The model under review builds one solid part; all positions refer to its coordinate system, in mm. A direction names the side the tool comes from. Coordinates: 2 decimals unless noted, no trailing zeros. Loops run counter-clockwise (first coordinate to the right, second up) from the corner with the lowest first, then second, coordinate; pieces in that order, holes last. Notation, with made-up numbers: (43, 37) - (65, 37) arc R29 ccw to (65, 74) - close; hole circle Ø2 at (60.5, 72). An arc over 180 degrees is marked (long way). Answer in a Markdown table with one row per item. Add a question column.
(1) We need section C-C on y = 63. Write out the cut boundary in (x, z), plus the area to 3 significant figures.
(2) Mouldability with a two-part tool opening along Y and no side actions: class faces 1 (the flat face through (-8.5, 32.2, -18)), 2 (the cylindrical face through (1.107, 43.353, -16.348)), 3 (the flat face through (0, 21.175, 22)), 4 (the cylindrical face through (-9, 59, 19)) as +Y half, -Y half, draft (parallel to the pull), parting line (faces both ways), or undercut.
(3) For P1, Ø9, axis at y = 60.42, z = -7.32, coming from the -X side; P2, Ø1.9, axis at x = -12.5, z = -17.5, coming from the +Y side (3 decimals); P3, Ø6, axis at x = 6.5, y = 22, coming from the +Z side; P4, Ø5, axis at x = 13.5, y = 33, coming from the +Z side, all flat-tipped, find the tip position at first contact; note any pin that passes through.
(4) For line 1 along Y through (x, z) = (-15.35, -17) (3 decimals); line 2 along Y through (x, z) = (-8, -3) (3 decimals); line 3 along Y through (x, z) = (1, 22) (3 decimals), list the stretches that pass through material, from the lowest coordinate up.
(5) We need section A-A on x = 15.35. Write out the cut boundary in (y, z) (3 decimals), plus the area to 3 significant figures.
(6) We need section D-D on z = 14. Write out the cut boundary in (x, y), plus the area to 3 significant figures.
(7) We need section B-B on y = 38. Write out the cut boundary in (x, z).
(8) Machinability: for faces 5 (the flat face through (-9, 35, -14.65)), 6 (the flat face through (0, 11, 21)), 7 (the flat face through (0, 59, 21)), which of the approach directions +Z, -Z, +X, -X, +Y, -Y give a long, thin tool a straight path to every point of the face, cutting with its end or side? Answer none if there is none.
from build123d import *

# Parameters (mm, degrees)
SKETCH1_W           = 20
SKETCH1_H           = 42
BOSS_EXTRUDE1_DEPTH = 69.85
FILLET1_R           = 5
SKETCH3_W           = 42
SKETCH3_H           = 42
BOSS_EXTRUDE2_DEPTH = 6.35
SKETCH4_W           = 16
SKETCH4_H           = 24
CUT_EXTRUDE2_DEPTH  = 80.252902155
SKETCH5_R           = 13
CUT_EXTRUDE3_DEPTH  = 3
CUT_EXTRUDE4_REACH  = 84.71
SKETCH7_R           = 8.5
SKETCH8_R           = 4
CUT_EXTRUDE5_DEPTH  = 80.252902155
FILLET2_R           = 6
FILLET3_R           = 4
FILLET4_R           = 3
SKETCH9_W           = 20
SKETCH9_H           = 27.5
BOSS_EXTRUDE3_DEPTH = 6.35
SKETCH2_R           = 7.5
CUT_EXTRUDE1_DEPTH  = 76.901399855
SKETCH10_W          = 20
SKETCH10_H          = 4
BOSS_EXTRUDE4_DEPTH = 5
FILLET6_R           = 3
SKETCH11_R          = 2
SKETCH11_R_2        = 1.5
CUT_EXTRUDE6_DEPTH  = 7


with BuildPart() as part:
    # Sketch1 → Boss-Extrude1 (new body)
    with BuildSketch(Plane(origin=(0, 0, 0), x_dir=(1, 0, 0), z_dir=(0, 1, 0))):
        Rectangle(SKETCH1_W, SKETCH1_H)
    extrude(amount=BOSS_EXTRUDE1_DEPTH)

    # Fillet1
    fillet1_edges = [part.edges().sort_by_distance(p)[0] for p in [
        (10, 34.925, 21),
        (-10, 34.925, 21),
    ]]
    fillet(fillet1_edges, radius=FILLET1_R)

    # Sketch3 → Boss-Extrude2 (add)
    with BuildSketch(Plane(origin=(0, 0, -21), x_dir=(-1, 0, 0), z_dir=(0, 0, -1))):
        with Locations((0, 34.925)):
            Rectangle(SKETCH3_W, SKETCH3_H)
    extrude(amount=-BOSS_EXTRUDE2_DEPTH)

    # Sketch4 → Cut-Extrude2 (cut, through all)
    with BuildSketch(Plane(origin=(10, 0, 0), x_dir=(0, 0, -1), z_dir=(1, 0, 0))):
        with Locations((6.65, 34.925)):
            Rectangle(SKETCH4_W, SKETCH4_H)
    extrude(amount=-CUT_EXTRUDE2_DEPTH, mode=Mode.SUBTRACT)

    # Sketch5 → Cut-Extrude3 (cut)
    with BuildSketch(Plane(origin=(0, 0, -21), x_dir=(-1, 0, 0), z_dir=(0, 0, -1))):
        with Locations((0, 34.925)):
            Circle(SKETCH5_R)
    extrude(amount=-CUT_EXTRUDE3_DEPTH, mode=Mode.SUBTRACT)

    # Sketch7 → Cut-Extrude4 (cut, up to next)
    with BuildSketch(Plane(origin=(0, 0, -18), x_dir=(-1, 0, 0), z_dir=(0, 0, -1)), mode=Mode.PRIVATE) as cut_extrude4_sk1:
        with Locations((0, 34.925)):
            Circle(SKETCH7_R)
    cut_extrude4_tool1 = extrude(cut_extrude4_sk1.sketch, amount=-CUT_EXTRUDE4_REACH, mode=Mode.PRIVATE) & part.part
    add(cut_extrude4_tool1.solids().sort_by_distance((0, 34.925, -18))[0], mode=Mode.SUBTRACT)

    # Sketch8 → Cut-Extrude5 (cut, through all)
    with BuildSketch(Plane(origin=(10, 0, 0), x_dir=(0, 0, -1), z_dir=(1, 0, 0))):
        with Locations((7.318215362, 60.425)):
            Circle(SKETCH8_R)
        with Locations((7.318215362, 9.425)):
            Circle(SKETCH8_R)
    extrude(amount=-CUT_EXTRUDE5_DEPTH, mode=Mode.SUBTRACT)

    # Fillet2
    fillet2_edges = [part.edges().sort_by_distance(p)[0] for p in [
        (0, 0, -21),
        (0, 69.85, -21),
    ]]
    fillet(fillet2_edges, radius=FILLET2_R)

    # Fillet3
    fillet3_edges = [part.edges().sort_by_distance(p)[0] for p in [
        (-21, 13.925, -17.825),
        (21, 55.925, -17.825),
        (-21, 55.925, -17.825),
        (21, 13.925, -17.825),
    ]]
    fillet(fillet3_edges, radius=FILLET3_R)

    # Fillet4
    fillet4_edges = [part.edges().sort_by_distance(p)[0] for p in [
        (0, 22.925, 1.35),
        (0, 46.925, -14.65),
        (0, 46.925, 1.35),
        (0, 22.925, -14.65),
    ]]
    fillet(fillet4_edges, radius=FILLET4_R)

    # Sketch9 → Boss-Extrude3 (add)
    with BuildSketch(Plane.XY.offset(21)):
        with Locations((0, 34.925)):
            Rectangle(SKETCH9_W, SKETCH9_H)
    extrude(amount=-BOSS_EXTRUDE3_DEPTH)

    # Sketch2 → Cut-Extrude1 (cut, through all)
    with BuildSketch(Plane(origin=(0, 69.85, 0), x_dir=(1, 0, 0), z_dir=(0, 1, 0))):
        with Locations(Location((0, -11.254449914, 0), (0, 0, 270))):
            Circle(SKETCH2_R)
    extrude(amount=-CUT_EXTRUDE1_DEPTH, mode=Mode.SUBTRACT)

    # Sketch10 → Boss-Extrude4 (add)
    with BuildSketch(Plane.XY.offset(21)):
        with Locations((0, 23.175)):
            Rectangle(SKETCH10_W, SKETCH10_H)
        with Locations((0, 46.675)):
            Rectangle(SKETCH10_W, SKETCH10_H)
    extrude(amount=BOSS_EXTRUDE4_DEPTH)

    # Fillet6
    fillet6_edges = [part.edges().sort_by_distance(p)[0] for p in [
        (0, 21.175, 26),
        (0, 48.675, 26),
    ]]
    fillet(fillet6_edges, radius=FILLET6_R)

    # Sketch11 → Cut-Extrude6 (cut)
    with BuildSketch(Plane(origin=(85.430800997, 34.822301654, -21), x_dir=(-1, 0, 0), z_dir=(0, 0, -1))):
        with Locations((70.080800997, 15.452698346)):
            Circle(SKETCH11_R)
        with Locations(Location((100.780800997, -15.247301654, 0), (0, 0, 180))):
            Circle(SKETCH11_R_2)
        with Locations((70.080800997, -15.247301654)):
            Circle(SKETCH11_R_2)
        with Locations(Location((100.780800997, 15.452698346, 0), (0, 0, 180))):
            Circle(SKETCH11_R)
    extrude(amount=-CUT_EXTRUDE6_DEPTH, mode=Mode.SUBTRACT)


solid = part.part
Outcome:
| question | item | result |
|---|---|---|
| 1 | outline | (-10, -21) - (10, -21) - (10, -10.38) - (-10, -10.38) - close; (-10, -4.26) - (10, -4.26) - (10, 16) arc R5 ccw to (5, 21) - (-5, 21) arc R5 ccw to (-10, 16) - close; hole circle Ø15 at (0, 11.25) |
| 1 | area | 530 mm² |
| 2 | face 1 | undercut |
| 2 | face 2 | undercut |
| 2 | face 3 | -Y half |
| 2 | face 4 | draft |
| 3 | P1 | x = -10 |
| 3 | P2 | y = 55.925 |
| 3 | P3 | z = 26 |
| 3 | P4 | z = -14.65 |
| 4 | line 1 | 13.925 to 18.075, 21.075 to 48.275, 52.275 to 55.925 |
| 4 | line 2 | 0 to 22.925, 46.925 to 69.85 |
| 4 | line 3 | 21.175 to 25.175, 44.675 to 48.675 |
| 5 | outline | (13.925, -21) - (18.075, -21) - (18.075, -14.65) - (13.925, -14.65) - close; (21.075, -21) - (48.275, -21) - (48.275, -14.65) - (21.075, -14.65) - close; (52.275, -21) - (55.925, -21) - (55.925, -14.65) - (52.275, -14.65) - close |
| 5 | area | 222 mm² |
| 6 | outline | (-10, 0) - (-6.98, 0) - (-6.98, 69.85) - (-10, 69.85) - close; (6.98, 0) - (10, 0) - (10, 69.85) - (6.98, 69.85) - close |
| 6 | area | 422 mm² |
| 7 | outline | (-21, -21) - (-12.63, -21) - (-12.63, -18) - (-7.92, -18) - (-7.92, -14.65) - (-21, -14.65) - close; (-10, 1.35) - (10, 1.35) - (10, 21) - (-10, 21) - close; (7.92, -18) - (12.63, -18) - (12.63, -21) - (21, -21) - (21, -14.65) - (7.92, -14.65) - close; hole circle Ø15 at (0, 11.25) |
| 8 | face 5 | none |
| 8 | face 6 | +Z, +X, -X, -Y |
| 8 | face 7 | +Z, +X, -X, +Y |
